```python
from build123d import *

# Parameters (mm, degrees)
SKETCH1_R                                        = 57.15
BOSS_EXTRUDE1_DEPTH                              = 6.35
SKETCH2_R                                        = 6.35
CUT_EXTRUDE1_DEPTH                               = 1
CUT_EXTRUDE1_DEPTH_BACK                          = 7.35
SKETCH3_R                                        = 57.15
SKETCH3_R_2                                      = 17.653
BOSS_EXTRUDE2_DEPTH                              = 6.35
ANNULUS_ENTRANCE_R                               = 3.175
CUT_EXTRUDE2_DEPTH                               = 1
CUT_EXTRUDE2_DEPTH_BACK                          = 13.7
CSK_FOR_1_4_FLAT_HEAD_MACHINE_SCREW1_D           = 6.5278
CSK_FOR_1_4_FLAT_HEAD_MACHINE_SCREW1_CSINK_D     = 12.8778
CSK_FOR_1_4_FLAT_HEAD_MACHINE_SCREW1_CSINK_ANGLE = 82
CIRPATTERN1_COUNT                                = 6
SKETCH11_R                                       = 10.16
SKETCH11_R_2                                     = 3.175
BOSS_EXTRUDE3_DEPTH                              = 7.62
F_1_4_NPT_TAPPED_HOLE3_AT_2_COUNT                = 2
F_1_4_NPT_TAPPED_HOLE3_AT_2_PITCH                = 49.493351826
F_1_4_NPT_TAPPED_HOLE3_AT_3_COUNT                = 2
F_1_4_NPT_TAPPED_HOLE3_AT_3_PITCH                = 49.493351826


with BuildPart() as part:
    # Sketch1 → Boss-Extrude1 (new body)
    with BuildSketch(Plane(origin=(0, 0, 0), x_dir=(1, 0, 0), z_dir=(0, 1, 0))):
        Circle(SKETCH1_R)
    extrude(amount=BOSS_EXTRUDE1_DEPTH)

    # Sketch2 → Cut-Extrude1 (cut, two sides)
    with BuildSketch(Plane(origin=(0, 6.35, 0), x_dir=(1, 0, 0), z_dir=(0, 1, 0))) as cut_extrude1_sk:
        Circle(SKETCH2_R)
    extrude(amount=CUT_EXTRUDE1_DEPTH, mode=Mode.SUBTRACT)
    extrude(cut_extrude1_sk.sketch, amount=-CUT_EXTRUDE1_DEPTH_BACK, mode=Mode.SUBTRACT)

    # Sketch3 → Boss-Extrude2 (add)
    with BuildSketch(Plane(origin=(0, 6.35, 0), x_dir=(1, 0, 0), z_dir=(0, 1, 0))):
        Circle(SKETCH3_R)
        Circle(SKETCH3_R_2, mode=Mode.SUBTRACT)
    extrude(amount=BOSS_EXTRUDE2_DEPTH)

    # Annulus Entrance → Cut-Extrude2 (cut, two sides)
    with BuildSketch(Plane(origin=(0, 12.7, 0), x_dir=(1, 0, 0), z_dir=(0, 1, 0))) as cut_extrude2_sk:
        with Locations((28.575, 0)):
            Circle(ANNULUS_ENTRANCE_R)
        with Locations((-14.2875, -24.746675913)):
            Circle(ANNULUS_ENTRANCE_R)
        with Locations((-14.2875, 24.746675913)):
            Circle(ANNULUS_ENTRANCE_R)
    extrude(amount=CUT_EXTRUDE2_DEPTH, mode=Mode.SUBTRACT)
    extrude(cut_extrude2_sk.sketch, amount=-CUT_EXTRUDE2_DEPTH_BACK, mode=Mode.SUBTRACT)

    # CSK for 1/4 Flat Head Machine Screw1 (through all)
    with Locations(Plane(origin=(0, 12.7, -45.72), x_dir=(0, 0, 1), z_dir=(0, 1, 0))):
        with Locations((0, 0)):
            csk_for_1_4_flat_head_machine_screw1 = CounterSinkHole(CSK_FOR_1_4_FLAT_HEAD_MACHINE_SCREW1_D / 2, CSK_FOR_1_4_FLAT_HEAD_MACHINE_SCREW1_CSINK_D / 2, counter_sink_angle=CSK_FOR_1_4_FLAT_HEAD_MACHINE_SCREW1_CSINK_ANGLE)

    # CirPattern1: CSK for 1/4 Flat Head Machine Screw1 ×6 about axis
    cirpattern1_axis = Axis((0, 0, 0), (0, 1, 0))
    for i in range(1, CIRPATTERN1_COUNT):
        add(csk_for_1_4_flat_head_machine_screw1.rotate(cirpattern1_axis, i * 360 / CIRPATTERN1_COUNT), mode=Mode.SUBTRACT)

    # Sketch11 → Boss-Extrude3 (add)
    with BuildSketch(Plane(origin=(0, 12.7, 0), x_dir=(1, 0, 0), z_dir=(0, 1, 0))):
        with Locations((-14.2875, 24.746675913)):
            Circle(SKETCH11_R)
        with Locations((-14.2875, 24.746675913)):
            Circle(SKETCH11_R_2, mode=Mode.SUBTRACT)
        with Locations((28.575, 0)):
            Circle(SKETCH11_R)
        with Locations((28.575, 0)):
            Circle(SKETCH11_R_2, mode=Mode.SUBTRACT)
        with Locations((-14.2875, -24.746675913)):
            Circle(SKETCH11_R)
        with Locations((-14.2875, -24.746675913)):
            Circle(SKETCH11_R_2, mode=Mode.SUBTRACT)
    extrude(amount=BOSS_EXTRUDE3_DEPTH)

    # Sketch13 → 1/4 NPT Tapped Hole3 (revolve, cut)
    with BuildSketch(Plane(origin=(-14.2875, 20.32, -24.746675913), x_dir=(0, 0, 1), z_dir=(1, 0, 0))):
        Polygon((0, 0), (0, 20.411147279), (5.5626, 17.0688), (5.5626, 10.0203), (6.335555425, 10.0203), (6.6298445, 0.191445196), (6.858, 0), align=None)
    f_1_4_npt_tapped_hole3 = revolve(axis=Axis((-14.2875, 26.67, -24.746675913), (0, -1, 0)), mode=Mode.SUBTRACT)

    # 1/4 NPT Tapped Hole3 at 2: 1/4 NPT Tapped Hole3 ×2
    with Locations(*[Vector(0.866025404, 0, 0.5) * (i * F_1_4_NPT_TAPPED_HOLE3_AT_2_PITCH) for i in range(1, F_1_4_NPT_TAPPED_HOLE3_AT_2_COUNT)]):
        add(f_1_4_npt_tapped_hole3, mode=Mode.SUBTRACT)

    # 1/4 NPT Tapped Hole3 at 3: 1/4 NPT Tapped Hole3 ×2
    with Locations(*[(0, 0, i * F_1_4_NPT_TAPPED_HOLE3_AT_3_PITCH) for i in range(1, F_1_4_NPT_TAPPED_HOLE3_AT_3_COUNT)]):
        add(f_1_4_npt_tapped_hole3, mode=Mode.SUBTRACT)


solid = part.part
```
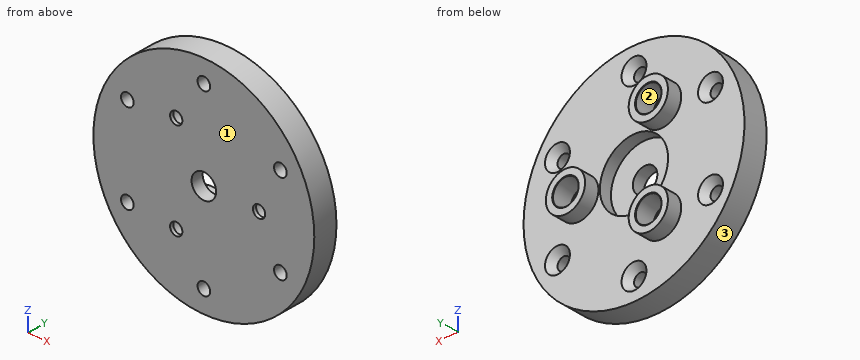
Read the model definition and answer for the solid it produces. Units are mm, in the model's axes. Face numbers are marked on the shaded views. Give positions to 0.01 mm unless a question says otherwise; leave off trailing zeros. Write each loop counter-clockwise with the first axis right and the second up, starting at its lowest first coordinate (ties: lowest second). Pieces come first, ordered by that corner, then holes. Notation, with made-up numbers: (52.25, -8.5) -> (59.25, -8.5) arc R15 ccw to (59.25, -2.5) -> close; hole circle Ø7 at (0, -29). An arc over 180 degrees is marked (long way). Answer in a Markdown table with one row per item.
1) Straight lines are drawn through the part: line 1 (Z direction, x = 0, y = 2.75); line 2 (X direction, y = 11, z = 25.5); line 3 (Z direction, x = 0.5, y = 11). For each, find the intervals that lie inside material, in ascending order. Write a range as [from, to].
Results list:
| item | result |
|---|---|
| line 1 | [-57.15, -48.98], [-42.46, -6.35], [6.35, 42.46], [48.98, 57.15] |
| line 2 | [-51.15, -43.8], [-35.39, -20.6], [-7.98, 35.39], [43.8, 51.15] |
| line 3 | [-57.15, -50.66], [-40.78, -17.65], [17.65, 40.78], [50.66, 57.15] |
2) Section D-D on x = 48.5 is taken. Give the vertices of the cut face in (y, z), plus the area to 3 significant figures.
Results list:
| item | result |
|---|---|
| outline | (0, -30.23) -> (12.7, -30.23) -> (12.7, 30.23) -> (0, 30.23) -> close |
| area | 768 mm^2 |
3) Section B-B on x = 0 is taken. Give the vertices of the cut face in (y, z), plus the area to 3 significant figures.
Results list:
| item | result |
|---|---|
| outline | (0, -57.15) -> (12.7, -57.15) -> (12.7, -52.16) -> (9.05, -48.98) -> (0, -48.98) -> close; (0, -42.46) -> (9.05, -42.46) -> (12.7, -39.28) -> (12.7, -17.65) -> (6.35, -17.65) -> (6.35, -6.35) -> (0, -6.35) -> close; (0, 6.35) -> (6.35, 6.35) -> (6.35, 17.65) -> (12.7, 17.65) -> (12.7, 39.28) -> (9.05, 42.46) -> (0, 42.46) -> close; (0, 48.98) -> (9.05, 48.98) -> (12.7, 52.16) -> (12.7, 57.15) -> (0, 57.15) -> close |
| area | 958 mm^2 |
4) Section C-C on y = 17.5 is taken. Give the vertices of the cut face in (x, z) (1 decimal), plus the area to 3 significant figures.
Results list:
| item | result |
|---|---|
| outline | circle Ø20.3 at (-14.3, -24.7); circle Ø20.3 at (-14.3, 24.7); circle Ø20.3 at (28.6, 0); hole circle Ø13.1 at (-14.3, -24.7); hole circle Ø13.1 at (-14.3, 24.7); hole circle Ø13.1 at (28.6, 0) |
| area | 568 mm^2 |
5) Section A-A on z = 45.72 is taken. Give the vertices of the cut face in (x, y).
Results list:
| item | result |
|---|---|
| outline | (-34.29, 0) -> (-3.26, 0) -> (-3.26, 9.05) -> (-6.44, 12.7) -> (-34.29, 12.7) -> close; (3.26, 0) -> (34.29, 0) -> (34.29, 12.7) -> (6.44, 12.7) -> (3.26, 9.05) -> close |
6) Determine the mould class of the marked faces 1, 2 and 3 for opening direction Z: released by +Z, released by -Z, zero draft, split by the parting line, or undercut.
Results list:
| item | result |
|---|---|
| face 1 | zero draft |
| face 2 | undercut |
| face 3 | split by the parting line |
7) Each of these flat-tipped pins is pushed along its axis until it touches: pin 1 Ø12 at (x, y) = (-42, 10.5) entering from -Z; pin 2 Ø10 at (x, z) = (-14.29, -24.75) entering from +Y; pin 3 Ø3 at (x, z) = (-25.5, -19) entering from +Y. Where does it stop, or does it pass through?
Results list:
| item | result |
|---|---|
| pin 1 | z = -44.39 |
| pin 2 | y = 2.92 |
| pin 3 | y = 12.7 |
